```python
from build123d import *

# Parameters (mm, degrees)
SKETCH1_W           = 38
SKETCH1_H           = 75
BOSS_EXTRUDE1_DEPTH = 4
SKETCH2_W           = 4
SKETCH2_H           = 19
CUT_EXTRUDE1_DEPTH  = 85.172442046


with BuildPart() as part:
    # Sketch1 → Boss-Extrude1 (new body)
    with BuildSketch(Plane(origin=(0, 0, 0), x_dir=(1, 0, 0), z_dir=(0, 1, 0))):
        with Locations((19, 37.5)):
            Rectangle(SKETCH1_W, SKETCH1_H)
    extrude(amount=BOSS_EXTRUDE1_DEPTH)

    # Sketch2 → Cut-Extrude1 (cut, through all)
    with BuildSketch(Plane(origin=(0, 4, 0), x_dir=(1, 0, 0), z_dir=(0, 1, 0))):
        Polygon((0, 0), (38, 0), (38, 25), (34, 25), (34, 6), (6, 6), (6, 25), (0, 25), align=None)
        Polygon((0, 50), (6, 50), (6, 69), (19, 69), (19, 75), (0, 75), align=None)
        with Locations((36, 59.5)):
            Rectangle(SKETCH2_W, SKETCH2_H)
    extrude(amount=-CUT_EXTRUDE1_DEPTH, mode=Mode.SUBTRACT)


solid = part.part
```
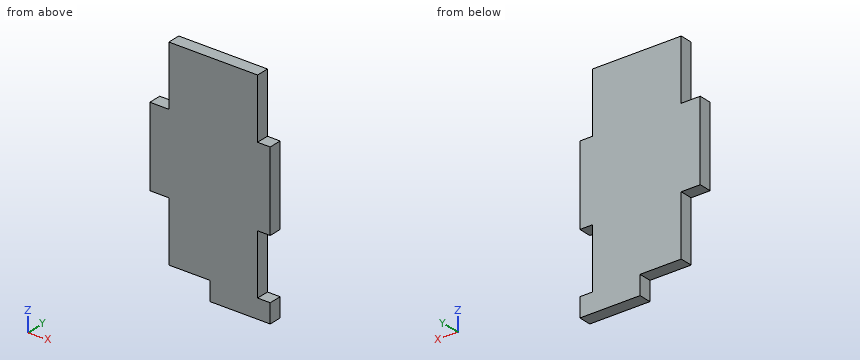
Input: part model. Units: mm. Frame: model coordinates. Round coordinates to 2 decimals unless told otherwise and drop trailing zeros. Loops run counter-clockwise (first coordinate to the right, second up) from the corner with the lowest first, then second, coordinate; pieces in that order, holes last. Notation, with made-up numbers: (-18.5, 66) -> (-0.5, 66) arc R35 ccw to (-0.5, 105) -> close; hole circle Ø7 at (10, 22). An arc over 180 degrees is marked (long way). Write each question's results on one line, items separated by ' | '.
1. Ray query, line 1 (Z direction, x = 35, y = 2.9); line 2 (X direction, y = 2, z = -65); line 3 (Z direction, x = 7.5, y = 3.5). Return the intervals inside material, ascending. Write a range as from..to.
Geometry results:
line 1: -75..-69, -50..-25 | line 2: 6..34 | line 3: -69..-6
2. Section A-A (y = 1.55). Return loops of the section in (x, z).
Geometry results:
outline: (0, -50) -> (6, -50) -> (6, -69) -> (19, -69) -> (19, -75) -> (38, -75) -> (38, -69) -> (34, -69) -> (34, -50) -> (38, -50) -> (38, -25) -> (34, -25) -> (34, -6) -> (6, -6) -> (6, -25) -> (0, -25) -> close
3. First-contact query: P1, Ø1.2, axis at x = 35.5, y = 2, coming from the +Z side; P2, Ø1.2, axis at y = 1.5, z = -13, coming from the -X side; P3, Ø2, axis at x = 14.5, y = 1, coming from the -Z side. Flat tips, straight axial feed; report the tip coordinate or a pass-through.
Geometry results:
P1: z = -25 | P2: x = 6 | P3: z = -69
4. Section C-C (x = 10). Return loops of the section in (y, z), and give its area (3 significant figures).
Geometry results:
outline: (0, -69) -> (4, -69) -> (4, -6) -> (0, -6) -> close | area: 252 mm2
5. Section B-B (z = -52). Return loops of the section in (x, y).
Geometry results:
outline: (6, 0) -> (34, 0) -> (34, 4) -> (6, 4) -> close
